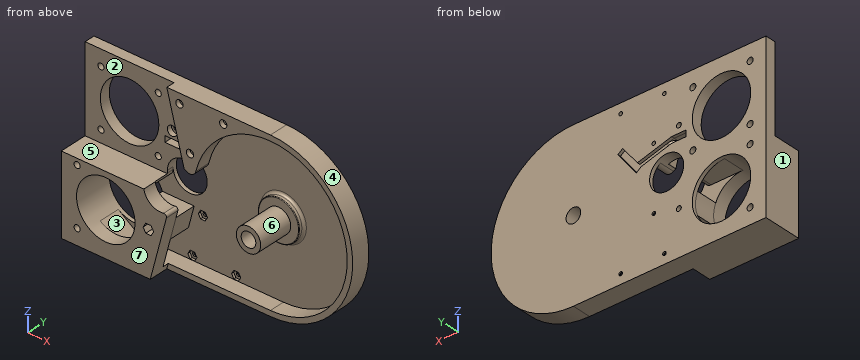
```python
from build123d import *

# Parameters (mm, degrees)
SALIENTE_EXTRUIR4_DEPTH    = 8.6
SALIENTE_EXTRUIR2_DEPTH    = 23
CORTAR_EXTRUIR1_DEPTH      = 174.347194959
CORTAR_EXTRUIR1_DEPTH_BACK = 174.347194959
CROQUIS2_R                 = 14
CROQUIS2_R_2               = 24
CROQUIS5_R                 = 2.5
CORTAR_EXTRUIR2_DEPTH      = 175.696336539
SALIENTE_EXTRUIR3_START    = -15.6
SALIENTE_EXTRUIR3_DEPTH    = 15.6
CORTAR_EXTRUIR3_DEPTH      = 174.347194959
CORTAR_EXTRUIR3_DEPTH_BACK = 174.347194959
CROQUIS7_R                 = 6
CORTAR_EXTRUIR4_DEPTH      = 5
CORTAR_EXTRUIR4_DEPTH_BACK = 12.5
REDONDEO1_R                = 2
CROQUIS9_R                 = 16.85
CROQUIS9_R_2               = 6
SALIENTE_EXTRUIR5_DEPTH    = 4.65
CROQUIS10_R                = 10
CROQUIS10_R_2              = 6
SALIENTE_EXTRUIR6_DEPTH    = 29
REDONDEO2_R                = 0.5
REDONDEO3_R                = 2
SALIENTE_EXTRUIR7_REACH    = 177.079
CROQUIS12_R                = 1.5
CORTAR_EXTRUIR5_DEPTH      = 174.111445318
CORTAR_EXTRUIR6_DEPTH      = 2
CROQUIS14_R                = 3
CORTAR_EXTRUIR7_DEPTH      = 3.7
CROQUIS15_R                = 2
CORTAR_EXTRUIR8_DEPTH      = 175.696336539
CROQUIS16_R                = 4
CORTAR_EXTRUIR9_DEPTH      = 4
CORTAR_EXTRUIR10_DEPTH     = 10
CORTAR_EXTRUIR11_DEPTH     = 2.5
CROQUIS20_W                = 12
CROQUIS20_H                = 5
CORTAR_EXTRUIR12_DEPTH     = 176.700917755
REDONDEO4_R                = 5


with BuildPart() as part:
    # Croquis1 → Saliente-Extruir4 (new body)
    with BuildSketch(Plane(origin=(0, 0, 0), x_dir=(1, 0, 0), z_dir=(0, 1, 0))):
        with BuildLine():
            Line((0, -67.5), (-158, -67.5))
            Line((-158, -67.5), (-158, 67.5))
            Line((-158, 67.5), (0, 67.5))
            ThreePointArc((0, 67.5), (67.5, 0), (0, -67.5))
        make_face()
    extrude(amount=SALIENTE_EXTRUIR4_DEPTH)

    # Croquis3 → Saliente-Extruir2 (add)
    with BuildSketch(Plane.XZ):
        Polygon((-85, -67.5), (-68.148148148, -2.5), (-158, -2.5), (-158, -67.5), align=None)
    extrude(amount=SALIENTE_EXTRUIR2_DEPTH)

    # Croquis2 → Cortar-Extruir1 (cut, two sides: drawn at the far end of the back side and taken through both)
    with BuildSketch(Plane(origin=(0, 0, 0), x_dir=(1, 0, 0), z_dir=(0, 1, 0)).offset(-CORTAR_EXTRUIR1_DEPTH_BACK)):
        with Locations(Location((-76.5, 0, 0), (0, 0, 66.051358792))):
            Circle(CROQUIS2_R)
        with Locations(Location((-121.5, 31, 0), (0, 0, 90))):
            Circle(CROQUIS2_R_2)
        with Locations(Location((-121.5, -31, 0), (0, 0, 90))):
            Circle(CROQUIS2_R_2)
    extrude(amount=CORTAR_EXTRUIR1_DEPTH + CORTAR_EXTRUIR1_DEPTH_BACK, mode=Mode.SUBTRACT)

    # Croquis5 → Cortar-Extruir2 (cut, through all)
    with BuildSketch(Plane(origin=(0, 8.6, 0), x_dir=(1, 0, 0), z_dir=(0, 1, 0))):
        with Locations(Location((-145, -7.5, 0), (0, 0, 270))):
            Circle(CROQUIS5_R)
        with Locations(Location((-145, -54.5, 0), (0, 0, 270))):
            Circle(CROQUIS5_R)
        with Locations(Location((-98, -54.5, 0), (0, 0, 270))):
            Circle(CROQUIS5_R)
        with Locations(Location((-98, -7.5, 0), (0, 0, 270))):
            Circle(CROQUIS5_R)
        with Locations(Location((-145, 7.5, 0), (0, 0, 270))):
            Circle(CROQUIS5_R)
        with Locations(Location((-145, 54.5, 0), (0, 0, 270))):
            Circle(CROQUIS5_R)
    extrude(amount=-CORTAR_EXTRUIR2_DEPTH, mode=Mode.SUBTRACT)

    # Croquis6 → Saliente-Extruir3 (add)
    with BuildSketch(Plane(origin=(0, 8.6, 0), x_dir=(1, 0, 0), z_dir=(0, 1, 0)).offset(SALIENTE_EXTRUIR3_START)):
        with BuildLine():
            Line((0, -67.5), (-85, -67.5))
            Line((-85, -67.5), (-70.817153658, -12.794735536))
            ThreePointArc((-70.817153658, -12.794735536), (-62.5, 0), (-70.817153658, 12.794735536))
            Line((-70.817153658, 12.794735536), (-85, 67.5))
            Line((-85, 67.5), (0, 67.5))
            ThreePointArc((0, 67.5), (67.5, 0), (0, -67.5))
        make_face()
    extrude(amount=SALIENTE_EXTRUIR3_DEPTH)

    # Croquis7 → Cortar-Extruir3 (cut, two sides: drawn at the far end of the back side and taken through both)
    with BuildSketch(Plane(origin=(0, 0, 0), x_dir=(1, 0, 0), z_dir=(0, 1, 0)).offset(-CORTAR_EXTRUIR3_DEPTH_BACK)):
        with Locations(Location((0, 0, 0), (0, 0, 270))):
            Circle(CROQUIS7_R)
    extrude(amount=CORTAR_EXTRUIR3_DEPTH + CORTAR_EXTRUIR3_DEPTH_BACK, mode=Mode.SUBTRACT)

    # Croquis8 → Cortar-Extruir4 (cut, two sides: drawn at the far end of the back side and taken through both)
    with BuildSketch(Plane.XZ.offset(7).offset(-CORTAR_EXTRUIR4_DEPTH_BACK)):
        with BuildLine():
            Line((0, -63), (-116.397014468, -63))
            ThreePointArc((-116.397014468, -63), (-117.923471798, -62.761294784), (-119.304179798, -62.067971208))
            Line((-119.304179798, -62.067971208), (-135.454393581, -50.526261798))
            ThreePointArc((-135.454393581, -50.526261798), (-144.354214963, -23.673004816), (-121.5, -7))
            Line((-121.5, -7), (-95.5, -7))
            ThreePointArc((-95.5, -7), (-91.964466094, -5.535533906), (-90.5, -2))
            Line((-90.5, -2), (-90.5, 0))
            ThreePointArc((-90.5, 0), (-84.130208097, 11.737969347), (-70.817153658, 12.794735536))
            ThreePointArc((-70.817153658, 12.794735536), (-69.810181657, 12.29822469), (-68.84623323, 11.722621474))
            ThreePointArc((-68.84623323, 11.722621474), (-64.266892893, 11.262463458), (-61.251513841, 14.739472589))
            ThreePointArc((-61.251513841, 14.739472589), (49.485284546, 38.989827051), (0, -63))
        make_face()
    extrude(amount=CORTAR_EXTRUIR4_DEPTH + CORTAR_EXTRUIR4_DEPTH_BACK, mode=Mode.SUBTRACT)


with BuildPart() as cortar_extruir4_kept_piece:
    # of the separate pieces the step leaves, the one the design keeps (cortar_extruir4_pieces_kept)
    add(part.part.solids().sort_by_distance((0, 8.6, 67.5))[0])

    # Redondeo1
    redondeo1_edges = [cortar_extruir4_kept_piece.edges().sort_by_distance(p)[0] for p in [
        (-70.817153658, -17.5, -12.794735536),
    ]]
    fillet(redondeo1_edges, radius=REDONDEO1_R)

    # Croquis9 → Saliente-Extruir5 (add)
    with BuildSketch(Plane.XZ.offset(-5.5)):
        with Locations(Location((0, 0, 0), (0, 0, 270))):
            Circle(CROQUIS9_R)
        with Locations(Location((0, 0, 0), (0, 0, 90))):
            Circle(CROQUIS9_R_2, mode=Mode.SUBTRACT)
    extrude(amount=SALIENTE_EXTRUIR5_DEPTH)

    # Croquis10 → Saliente-Extruir6 (add)
    with BuildSketch(Plane.XZ.offset(-0.85)):
        with Locations(Location((0, 0, 0), (0, 0, 90))):
            Circle(CROQUIS10_R)
        with Locations(Location((0, 0, 0), (0, 0, 90))):
            Circle(CROQUIS10_R_2, mode=Mode.SUBTRACT)
    extrude(amount=SALIENTE_EXTRUIR6_DEPTH)

    # Redondeo2
    redondeo2_edges = [cortar_extruir4_kept_piece.edges().sort_by_distance(p)[0] for p in [
        (0, 0.85, 16.85),
    ]]
    fillet(redondeo2_edges, radius=REDONDEO2_R)

    # Redondeo3
    redondeo3_edges = [cortar_extruir4_kept_piece.edges().sort_by_distance(p)[0] for p in [
        (0, 5.5, 16.85),
    ]]
    fillet(redondeo3_edges, radius=REDONDEO3_R)

    # Croquis11 → Saliente-Extruir7 (add, up to next)
    with BuildSketch(Plane.XZ.offset(-5.5), mode=Mode.PRIVATE) as saliente_extruir7_sk1:
        with BuildLine():
            Line((-73.203703704, -22), (-77.87037037, -40))
            Line((-77.87037037, -40), (-99.251404539, -40))
            ThreePointArc((-99.251404539, -40), (-97.5, -31), (-99.251404539, -22))
            Line((-99.251404539, -22), (-73.203703704, -22))
        make_face()
    saliente_extruir7_tool1 = extrude(saliente_extruir7_sk1.sketch, amount=SALIENTE_EXTRUIR7_REACH, mode=Mode.PRIVATE) - cortar_extruir4_kept_piece.part
    add(saliente_extruir7_tool1.solids().sort_by_distance((-86.771742, 5.5, -30.689413))[0])

    # Croquis12 → Cortar-Extruir5 (cut, through all)
    with BuildSketch(Plane.XZ.offset(7)):
        with Locations(Location((-74.661436633, 59.5, 0), (0, 0, 270))):
            Circle(CROQUIS12_R)
        with Locations(Location((-66.012679429, 26.140507926, 0), (0, 0, 270))):
            Circle(CROQUIS12_R)
        with Locations(Location((-38.73951471, 59.5, 0), (0, 0, 270))):
            Circle(CROQUIS12_R)
        with Locations(Location((-38.73951471, -59.5, 0), (0, 0, 270))):
            Circle(CROQUIS12_R)
        with Locations(Location((-74.661436633, -59.5, 0), (0, 0, 270))):
            Circle(CROQUIS12_R)
        with Locations(Location((-66.012679429, -26.140507926, 0), (0, 0, 270))):
            Circle(CROQUIS12_R)
    extrude(amount=-CORTAR_EXTRUIR5_DEPTH, mode=Mode.SUBTRACT)

    # Croquis13 → Cortar-Extruir6 (cut)
    with BuildSketch(Plane.XZ.offset(-5.5)):
        Polygon((-70.908659884, -59.5), (-72.785048259, -56.25), (-76.537825008, -56.25), (-78.414213383, -59.5), (-76.537825008, -62.75), (-72.785048259, -62.75), align=None)
        Polygon((-62.259902679, -26.140507926), (-64.136291054, -22.890507926), (-67.889067804, -22.890507926), (-69.765456179, -26.140507926), (-67.889067804, -29.390507926), (-64.136291054, -29.390507926), align=None)
        Polygon((-34.986737961, -59.5), (-36.863126336, -56.25), (-40.615903085, -56.25), (-42.49229146, -59.5), (-40.615903085, -62.75), (-36.863126336, -62.75), align=None)
    extrude(amount=-CORTAR_EXTRUIR6_DEPTH, mode=Mode.SUBTRACT)

    # Croquis14 → Cortar-Extruir7 (cut)
    with BuildSketch(Plane.XZ.offset(7)):
        with Locations(Location((-66.012679429, 26.140507926, 0), (0, 0, 270))):
            Circle(CROQUIS14_R)
        with Locations(Location((-74.661436633, 59.5, 0), (0, 0, 270))):
            Circle(CROQUIS14_R)
        with Locations(Location((-38.73951471, 59.5, 0), (0, 0, 270))):
            Circle(CROQUIS14_R)
    extrude(amount=-CORTAR_EXTRUIR7_DEPTH, mode=Mode.SUBTRACT)

    # Croquis15 → Cortar-Extruir8 (cut, through all)
    with BuildSketch(Plane.XZ.offset(23)):
        with Locations(Location((-86.518518519, -31, 0), (0, 0, 270))):
            Circle(CROQUIS15_R)
        with Locations(Location((-86.518518519, 31, 0), (0, 0, 90))):
            Circle(CROQUIS15_R)
    extrude(amount=-CORTAR_EXTRUIR8_DEPTH, mode=Mode.SUBTRACT)

    # Croquis16 → Cortar-Extruir9 (cut)
    with BuildSketch(Plane.XZ):
        with Locations(Location((-86.518518519, 31, 0), (0, 0, 270))):
            Circle(CROQUIS16_R)
    extrude(amount=-CORTAR_EXTRUIR9_DEPTH, mode=Mode.SUBTRACT)

    # Croquis17 → Cortar-Extruir10 (cut)
    with BuildSketch(Plane.XZ.offset(23)):
        Polygon((-82.1883915, -31), (-84.353455009, -27.25), (-88.683582028, -27.25), (-90.848645537, -31), (-88.683582028, -34.75), (-84.353455009, -34.75), align=None)
    extrude(amount=-CORTAR_EXTRUIR10_DEPTH, mode=Mode.SUBTRACT)

    # Croquis19 → Cortar-Extruir11 (cut)
    with BuildSketch(Plane(origin=(0, 8.6, 0), x_dir=(1, 0, 0), z_dir=(0, 1, 0))):
        Polygon((-52.482988664, -17.255771853), (-40.471682692, -33.003928572), (-36.496071428, -29.971682692), (-51.657300826, -10.09362637), (-55.63291209, -13.12587225), (-80.518518519, -20), (-92.518518519, -20), (-92.518518519, -25), (-80.518518519, -25), align=None)
    extrude(amount=-CORTAR_EXTRUIR11_DEPTH, mode=Mode.SUBTRACT)

    # Croquis20 → Cortar-Extruir12 (cut, through all)
    with BuildSketch(Plane(origin=(0, 8.6, 0), x_dir=(1, 0, 0), z_dir=(0, 1, 0))):
        with Locations((-86.518518519, -22.5)):
            Rectangle(CROQUIS20_W, CROQUIS20_H)
    extrude(amount=-CORTAR_EXTRUIR12_DEPTH, mode=Mode.SUBTRACT)

    # Redondeo4
    # the kernel refuses this fillet: 5 mm, written as the material it takes off along each edge
    with BuildSketch(Plane(origin=(-80.518518519, 6.1, 25), x_dir=(0, -1, 0), z_dir=(0, 0, -1))) as redondeo4_piece_1_section:
        with BuildLine():
            CenterArc((REDONDEO4_R, -REDONDEO4_R), REDONDEO4_R, 90, 90)
            Line((0, -REDONDEO4_R), (0, 0))
            Line((0, 0), (REDONDEO4_R, 0))
        make_face()
    redondeo4_piece_1 = extrude(amount=5, mode=Mode.PRIVATE)
    redondeo4_piece_1 = split(redondeo4_piece_1, bisect_by=Plane(origin=(-78.850583618, 4.928175606, 24.539267905), z_dir=(-0.26625771274306737, 0, -0.9639018779963188)), keep=Keep.TOP, mode=Mode.PRIVATE)
    redondeo4_piece_1 = split(redondeo4_piece_1, bisect_by=Plane(origin=(-80.133815165, 4.928175606, 19.893733753), z_dir=(0.2662577127430677, 0, 0.9639018779963188)), keep=Keep.TOP, mode=Mode.PRIVATE)
    add(redondeo4_piece_1, mode=Mode.SUBTRACT)
    with BuildSketch(Plane(origin=(-80.518518519, 6.1, 25), x_dir=(0, -1, 0), z_dir=(0, 0, -1))) as redondeo4_piece_2_section:
        with BuildLine():
            CenterArc((REDONDEO4_R, -REDONDEO4_R), REDONDEO4_R, 90, 90)
            Line((0, -REDONDEO4_R), (0, 0))
            Line((0, 0), (REDONDEO4_R, 0))
        make_face()
    redondeo4_piece_2 = extrude(amount=17.5, mode=Mode.PRIVATE)
    redondeo4_piece_2 = split(redondeo4_piece_2, bisect_by=Plane(origin=(-78.44415934, 5.567637436, 19.427001708), z_dir=(0.2662577127430677, 0, 0.9639018779963188)), keep=Keep.TOP, mode=Mode.PRIVATE)
    redondeo4_piece_2 = split(redondeo4_piece_2, bisect_by=Plane(origin=(-78.36792826, 5.567637436, 20), z_dir=(0, 0, -1)), keep=Keep.TOP, mode=Mode.PRIVATE)
    add(redondeo4_piece_2, mode=Mode.SUBTRACT)


solid = cortar_extruir4_kept_piece.part
```
Input: part model. Units: mm. Frame: model coordinates. Face numbers are marked on the shaded views. A direction names the side the tool comes from. Coordinates: 2 decimals unless noted, no trailing zeros. Write each loop counter-clockwise with the first axis right and the second up, starting at its lowest first coordinate (ties: lowest second). Pieces come first, ordered by that corner, then holes. Notation, with made-up numbers: (54, 61.5) - (103, 61.5) arc R29 ccw to (103, 98.5) - close; hole circle Ø8 at (31.25, 45.25). An arc over 180 degrees is marked (long way). Put each result on its own line as item: value. Start each with the question number.
1) Mould query, pull axis X, two halves, no side actions, for the marked faces 1, 2, 3 and 4. Classes: pulls with the +X half, pulls with the -X half, needs draft (parallel to the pull), parting line crosses it, or undercut.
2) Cut plane C-C (x = 29.5). Return the cut outline in (y, z).
3) Cut plane A-A (y = -17.5). Return the cut outline in (x, z).
4) Contact query for flat-ended pins moving along their axis: pin 1 (5 mm diameter, centred on x = -38.5, z = -59, fed in from -Y); pin 2 (3 mm diameter, centred on x = -73.5, z = 60, fed in from -Y); pin 3 (1.5 mm diameter, centred on x = -97, y = -6.5, fed in from +Z); pin 4 (6 mm diameter, centred on y = -12.5, z = 14.5, fed in from -X). Output: stop coordinate, or through.
5) Reachability of the marked faces 5, 6 and 7 from +Z, -Z, +X, -X, +Y, -Y: full face, straight path, thin tool, end or side. Return the list, or none.
6) Cut plane D-D (x = -138.5). Return the cut outline in (y, z).
7) Cut plane B-B (x = -106.5). Return the cut outline in (y, z) (3 decimals).
8) Ray query, L1, parallel to Z at x = -121, y = 6; L2, parallel to X at y = -1, z = 0; L3, parallel to X at y = 2, z = -26.5. Return the intervals inside material, ascending.
Resolved:
1. face 1: pulls with the -X half
1. face 2: needs draft
1. face 3: undercut
1. face 4: pulls with the +X half
2. outline: (-7, -60.71) - (8.6, -60.71) - (8.6, 60.71) - (-7, 60.71) - (-7, 55.67) - (5.5, 55.67) - (5.5, -55.67) - (-7, -55.67) - close
3. outline: (-158, -67.5) - (-85, -67.5) - (-71.71, -16.25) arc R2 ccw to (-74, -13.78) arc R14 cw to (-90.27, -2.5) - (-158, -2.5) - close; circle Ø20 at (0, 0); hole circle Ø5 at (-145, -54.5); hole circle Ø5 at (-145, -7.5); hole circle Ø48 at (-121.5, -31); hole (-90.85, -31) - (-88.68, -34.75) - (-84.35, -34.75) - (-82.19, -31) - (-84.35, -27.25) - (-88.68, -27.25) - close; hole circle Ø12 at (0, 0)
4. pin 1: stops at y = 7.5
4. pin 2: stops at y = -3.3
4. pin 3: stops at z = -2.5
4. pin 4: passes through
5. face 5: +Z, -X, -Y
5. face 6: -Y
5. face 7: +Z, -Z, -X, -Y
6. outline: (-23, -67.5) - (8.6, -67.5) - (8.6, -47.94) - (-23, -47.94) - close; (-23, -14.06) - (8.6, -14.06) - (8.6, 14.06) - (0, 14.06) - (0, -2.5) - (-23, -2.5) - close; (0, 47.94) - (8.6, 47.94) - (8.6, 67.5) - (0, 67.5) - close
7. outline: (-23, -67.5) - (8.6, -67.5) - (8.6, -49.735) - (5.5, -49.735) - (5.5, -63) - (-12, -63) - (-12, -49.735) - (-23, -49.735) - close; (-23, -12.265) - (-12, -12.265) - (-12, -7) - (5.5, -7) - (5.5, -12.265) - (8.6, -12.265) - (8.6, 12.265) - (0, 12.265) - (0, -2.5) - (-23, -2.5) - close; (0, 49.735) - (8.6, 49.735) - (8.6, 67.5) - (0, 67.5) - close
8. L1: z = -67.5 to -54.99, -7.01 to 7.01, 54.99 to 67.5
8. L2: x = -10 to -6, 6 to 10, 63 to 67.5
8. L3: x = -158 to -145.07, -97.93 to -74.37, 57.16 to 62.08
